Job drawing, mm, ordinate dimensions from the low corner. One solid piece. A direction names the side the tool comes from. Give positions to 0.01 mm unless a question says otherwise; leave off trailing zeros. Order: outer loops, then holes, each group sorted by start corner. A loop starts at its lowest first (then second) coordinate and runs counter-clockwise, first axis right, second up. Notation, with made-up numbers: (-38.5, 63) - (-6.5, 63) arc R4 cw to (-6.5, 70) - close; hole circle Ø8 at (11, 81). An arc over 180 degrees is marked (long way). Use one line per item in the form item = value. Start each with the question number.
1. Band-saw the part on B-B, the plane x = 5.5. List the corners of the cut face in (y, z) (3 decimals).
2. Drill centre lines: line 1 (X direction, y = 6, z = 2.25) (3 decimals); line 2 (Y direction, x = 5.25, z = 2.95) (3 decimals). Where is each one in solid material? Low to high.
3. Band-saw the part on C-C, the plane z = 1. List the corners of the cut face in (x, y) (3 decimals), plus the area to 3 significant figures.
4. Tool access for the marked faces 1 and 2: list every direction of +Z, -Z, +X, -X, +Y, -Y with a clear straight run to the whole face (end or side of a thin tool).
5. Pin check, flat tip, straight feed: P1, Ø1.5, axis at x = 7.5, z = 3, coming from the -Y side. Stop position of the tip, or through.
6. Pull direction X, two halves, no side cores. Call the marked faces 3, 4 and 5: +X half, -X half, draft (parallel to the pull), parting line (faces both ways), or undercut.
7. Band-saw the part on A-A, the plane y = 3.5. List the corners of the cut face in (x, z) (3 decimals).
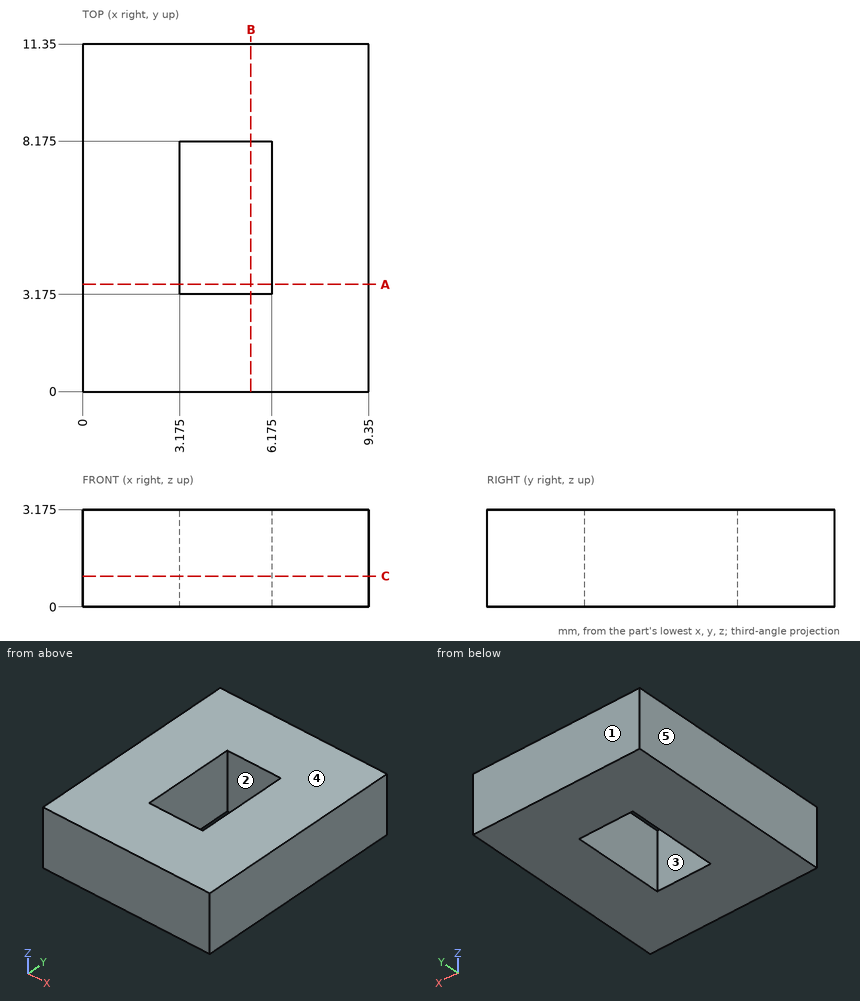
From the geometry:
q1.outline = (0, 0) - (3.175, 0) - (3.175, 3.175) - (0, 3.175) - close; (8.175, 0) - (11.35, 0) - (11.35, 3.175) - (8.175, 3.175) - close
q2.line_1 = 0 to 3.175, 6.175 to 9.35
q2.line_2 = 0 to 3.175, 8.175 to 11.35
q3.outline = (0, 0) - (9.35, 0) - (9.35, 11.35) - (0, 11.35) - close; hole (3.175, 3.175) - (6.175, 3.175) - (6.175, 8.175) - (3.175, 8.175) - close
q3.area = 91.1 mm²
q4.face_1 = +Z, -Z, +X, -X, +Y
q4.face_2 = +Z, -Z
q5.P1 = 0
q6.face_3 = undercut
q6.face_4 = draft
q6.face_5 = -X half
q7.outline = (0, 0) - (3.175, 0) - (3.175, 3.175) - (0, 3.175) - close; (6.175, 0) - (9.35, 0) - (9.35, 3.175) - (6.175, 3.175) - close
